from build123d import *

# Parameters (mm, degrees)
SKETCH1_W               = 58.166
SKETCH1_H               = 73.439999932
BOSS_EXTRUDE1_DEPTH     = 5.08
SKETCH2_W               = 27.686
SKETCH2_H               = 5.08
CUT_EXTRUDE1_DEPTH      = 94.821764778
CUT_EXTRUDE2_DEPTH      = 94.821764778
CUT_EXTRUDE2_DEPTH_BACK = 94.821764778
SKETCH7_R               = 16.51
FILLET2_R               = 21.59
FILLET3_R               = 12.7


with BuildPart() as part:
    # Sketch1 → Boss-Extrude1 (new body)
    with BuildSketch(Plane.XY):
        with Locations((29.083, 36.719999966)):
            Rectangle(SKETCH1_W, SKETCH1_H)
    extrude(amount=BOSS_EXTRUDE1_DEPTH)

    # Sketch2 → Cut-Extrude1 (cut, through all)
    with BuildSketch(Plane.XY.offset(5.08)):
        with Locations((29.083, 65.819999932)):
            Rectangle(SKETCH2_W, SKETCH2_H)
    extrude(amount=-CUT_EXTRUDE1_DEPTH, mode=Mode.SUBTRACT)

    # Sketch7 → Cut-Extrude2 (cut, two sides: drawn at the far end of the back side and taken through both)
    with BuildSketch(Plane.XY.offset(5.08).offset(-CUT_EXTRUDE2_DEPTH_BACK)):
        with Locations((29.099999966, 29.1)):
            Circle(SKETCH7_R)
    extrude(amount=CUT_EXTRUDE2_DEPTH + CUT_EXTRUDE2_DEPTH_BACK, mode=Mode.SUBTRACT)

    # Fillet2
    fillet2_edges = [part.edges().sort_by_distance(p)[0] for p in [
        (58.166, 0, 2.54),
        (0, 0, 2.54),
    ]]
    fillet(fillet2_edges, radius=FILLET2_R)

    # Fillet3
    fillet3_edges = [part.edges().sort_by_distance(p)[0] for p in [
        (0, 73.439999932, 2.54),
        (58.166, 73.439999932, 2.54),
    ]]
    fillet(fillet3_edges, radius=FILLET3_R)


solid = part.part
Design review of the part built by this model. Coordinates are the model's own, in mm. A direction names the side the tool comes from. Give positions to 0.01 mm unless a question says otherwise; leave off trailing zeros. Order: outer loops, then holes, each group sorted by start corner. A loop starts at its lowest first (then second) coordinate and runs counter-clockwise, first axis right, second up. Notation, with made-up numbers: (55, 78.25) - (89, 78.25) arc R28 ccw to (89, 117.25) - close; hole circle Ø1 at (39, 10.5). An arc over 180 degrees is marked (long way). Use CSV: the item, a comma, the result in double quotes. Start each with the question number.
Q1. Draft analysis for pull direction X (two halves, no side actions). For faces 1 (the face through (29, 63.28, 3)), 2 (the face through (51.674, 6.157, 2.576)), 3 (the face through (29, 73.44, 3)), 4 (the face through (42.926, 66, 3)), state which applies: pulls with the +X half, pulls with the -X half, needs draft (parallel to the pull), parting line crosses it, or undercut.
Q2. For P1, Ø3, axis at x = 26, y = 43, coming from the +Z side; P2, Ø10, axis at x = 8, y = 21.5, coming from the -Z side; P3, Ø2.5, axis at y = 65.5, z = 3.5, coming from the -X side, all flat-tipped, find the tip position at first contact; note any pin that passes through.
Q3. For line 1 (Y direction, x = 29.1, z = 4); line 2 (X direction, y = 29.1, z = 2.3); line 3 (Y direction, x = 16.5, z = 2.6), list the stretches that pass through material, from the lowest coordinate up.
Q4. Take a section at A-A (x = 29.1). State the section outline as (y, z) points, and give its area (3 significant figures).
Q5. Take a section at C-C (z = 2). State the section outline as (x, y) points, and give its area (3 significant figures).
Q6. Machinability: for faces 5 (the face through (29, 0, 3)), 6 (the face through (15.24, 66, 3)), which of the approach directions +Z, -Z, +X, -X, +Y, -Y give a long, thin tool a straight path to every point of the face, cutting with its end or side? Answer none if there is none.
Q7. Take a section at D-D (x = 14). State the section outline as (y, z) points.
Q8. Take a section at B-B (y = 29.1). State the section outline as (x, z) points.
Calculated:
1,face 1,"undercut"
1,face 2,"pulls with the +X half"
1,face 3,"needs draft"
1,face 4,"undercut"
2,P1,"passes through"
2,P2,"stops at z = 0"
2,P3,"stops at x = 0.49"
3,line 1,"y = 0 to 12.59, 45.61 to 63.28, 68.36 to 73.44"
3,line 2,"x = 0 to 12.59, 45.61 to 58.17"
3,line 3,"y = 0.61 to 18.43, 39.77 to 63.28, 68.36 to 73.44"
4,outline,"(0, 0) - (12.59, 0) - (12.59, 5.08) - (0, 5.08) - close; (45.61, 0) - (63.28, 0) - (63.28, 5.08) - (45.61, 5.08) - close; (68.36, 0) - (73.44, 0) - (73.44, 5.08) - (68.36, 5.08) - close"
4,area,"180 mm²"
5,outline,"(0, 21.59) arc R21.59 ccw to (21.59, 0) - (36.58, 0) arc R21.59 ccw to (58.17, 21.59) - (58.17, 60.74) arc R12.7 ccw to (45.47, 73.44) - (12.7, 73.44) arc R12.7 ccw to (0, 60.74) - close; hole circle Ø33.02 at (29.1, 29.1); hole (15.24, 63.28) - (42.93, 63.28) - (42.93, 68.36) - (15.24, 68.36) - close"
5,area,"3,010 mm²"
6,face 5,"+Z, -Z, +X, -X, -Y"
6,face 6,"+Z, -Z"
7,outline,"(1.38, 0) - (22.42, 0) - (22.42, 5.08) - (1.38, 5.08) - close; (35.78, 0) - (73.44, 0) - (73.44, 5.08) - (35.78, 5.08) - close"
8,outline,"(0, 0) - (12.59, 0) - (12.59, 5.08) - (0, 5.08) - close; (45.61, 0) - (58.17, 0) - (58.17, 5.08) - (45.61, 5.08) - close"
